```python
from build123d import *


with BuildPart() as f1:
    # F0 (on Front) → F1 (revolve)
    with BuildSketch(Plane.XZ):
        with BuildLine():
            Line((0, -59.163861), (14.661524, -59.163861))
            ThreePointArc((14.661524, -59.163861), (27.786311, -40.224746), (29.719422, -17.263623))
            ThreePointArc((29.719422, -17.263623), (18.366684, 2.688503), (17.28029, 25.618652))
            Line((17.28029, 25.618652), (0, 25.618652))
            Line((0, 25.618652), (0, -59.163861))
        make_face()
    revolve(axis=Axis((0, 0, -16.772605), (0, 0, 1)))

    # F2 (on Front) → F3 (revolve, cut)
    with BuildSketch(Plane.XZ):
        with BuildLine():
            Line((0, 25.88696), (-11.040121, 25.88696))
            Line((-11.040121, 25.88696), (-20.404007, -17.464366))
            ThreePointArc((-20.404007, -17.464366), (-20.462926, -36.483582), (-12.774174, -53.879477))
            Line((-12.774174, -53.879477), (0, -53.879477))
            Line((0, -53.879477), (0, 25.88696))
        make_face()
    revolve(axis=Axis((0, 0, -13.996258), (0, 0, -1)), mode=Mode.SUBTRACT)


solid = f1.part
```
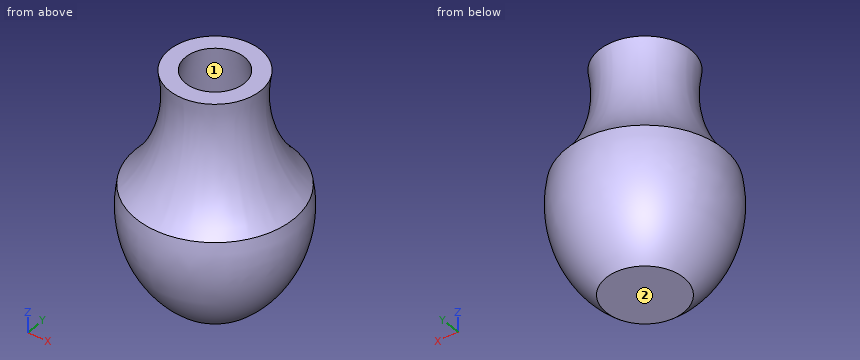
For this review, take the finished solid that the model builds, in its own axes (mm). Face numbers are marked on the shaded views. Round coordinates to 2 decimals unless told otherwise and drop trailing zeros. Order: outer loops, then holes, each group sorted by start corner. A loop starts at its lowest first (then second) coordinate and runs counter-clockwise, first axis right, second up.
Q1. Insertion check: P1, Ø3, axis at x = 4.5, y = 23.5, coming from the +Z side; P2, Ø12, axis at x = -12.5, z = -38, coming from the -Y side; P3, Ø2, axis at x = 15.5, y = 2.5, coming from the -Z side. Each pin has a flat end and moves straight along its axis. Give the tip position at first contact, or say it passes through.
Findings below:
P1: stops at z = -7.17
P2: stops at y = -28.42
P3: stops at z = -59.13
Q2. We need section A-A, the plane z = 12. Give the boundary of the cut face in (x, y).
Findings below:
outline: circle Ø33.23 at (0, 0); hole circle Ø28.08 at (0, 0)
Q3. Mouldability with a two-part tool opening along Y and no side actions: class the marked faces 1 and 2 as pulls with the +Y half, pulls with the -Y half, needs draft (parallel to the pull), parting line crosses it, or undercut.
Findings below:
face 1: undercut
face 2: needs draft
Q4. Wall thickness on line 1 (Y direction, x = -4, z = -7); line 2 (X direction, y = 12.5, z = -39); line 3 (X direction, y = 2.5, z = -14.5): over which ranges is each line inside the solid? List them lowest first.
Findings below:
line 1: y = -21.97 to -17.7, 17.7 to 21.97
line 2: x = -25.29 to -15.43, 15.43 to 25.29
line 3: x = -27.2 to -19.6, 19.6 to 27.2
